from build123d import *

# Parameters (mm, degrees)
CROQUIS1_R              = 4.1
SALIENTE_EXTRUIR1_DEPTH = 0.75


with BuildPart() as part:
    # Croquis1 → Saliente-Extruir1 (new, symmetric)
    with BuildSketch(Plane(origin=(0, 0, 0), x_dir=(1, 0, 0), z_dir=(0, 1, 0))):
        with Locations(Location((0, 0, 0), (0, 0, 270))):
            Circle(CROQUIS1_R)
        with BuildLine():
            Line((1.724717498, -2.212701665), (2.778614602, -0.387298335))
            ThreePointArc((2.778614602, -0.387298335), (2.890446656, -0.263302793), (3.043155854, -0.195766112))
            ThreePointArc((3.043155854, -0.195766112), (3.2022214, 0), (3.043155854, 0.195766112))
            ThreePointArc((3.043155854, 0.195766112), (2.890446656, 0.263302793), (2.778614602, 0.387298335))
            Line((2.778614602, 0.387298335), (1.724717498, 2.212701665))
            ThreePointArc((1.724717498, 2.212701665), (1.673250235, 2.371548836), (1.691116353, 2.537567222))
            ThreePointArc((1.691116353, 2.537567222), (1.6011107, 2.773205081), (1.352039501, 2.733333333))
            ThreePointArc((1.352039501, 2.733333333), (1.217196421, 2.634851628), (1.053897104, 2.6))
            Line((1.053897104, 2.6), (-1.053897104, 2.6))
            ThreePointArc((-1.053897104, 2.6), (-1.217196421, 2.634851628), (-1.352039501, 2.733333333))
            ThreePointArc((-1.352039501, 2.733333333), (-1.6011107, 2.773205081), (-1.691116353, 2.537567222))
            ThreePointArc((-1.691116353, 2.537567222), (-1.673250235, 2.371548836), (-1.724717498, 2.212701665))
            Line((-1.724717498, 2.212701665), (-2.778614602, 0.387298335))
            ThreePointArc((-2.778614602, 0.387298335), (-2.890446656, 0.263302793), (-3.043155854, 0.195766112))
            ThreePointArc((-3.043155854, 0.195766112), (-3.2022214, 0), (-3.043155854, -0.195766112))
            ThreePointArc((-3.043155854, -0.195766112), (-2.890446656, -0.263302793), (-2.778614602, -0.387298335))
            Line((-2.778614602, -0.387298335), (-1.724717498, -2.212701665))
            ThreePointArc((-1.724717498, -2.212701665), (-1.673250235, -2.371548836), (-1.691116353, -2.537567222))
            ThreePointArc((-1.691116353, -2.537567222), (-1.6011107, -2.773205081), (-1.352039501, -2.733333333))
            ThreePointArc((-1.352039501, -2.733333333), (-1.217196421, -2.634851628), (-1.053897104, -2.6))
            Line((-1.053897104, -2.6), (1.053897104, -2.6))
            ThreePointArc((1.053897104, -2.6), (1.217196421, -2.634851628), (1.352039501, -2.733333333))
            ThreePointArc((1.352039501, -2.733333333), (1.6011107, -2.773205081), (1.691116353, -2.537567222))
            ThreePointArc((1.691116353, -2.537567222), (1.673250235, -2.371548836), (1.724717498, -2.212701665))
        make_face(mode=Mode.SUBTRACT)
    extrude(amount=SALIENTE_EXTRUIR1_DEPTH, both=True)


solid = part.part
CAD build for the part. Positions are in the model's coordinates, mm. A direction names the side the tool comes from. Give positions to 0.01 mm unless a question says otherwise; leave off trailing zeros. Write each loop counter-clockwise with the first axis right and the second up, starting at its lowest first coordinate (ties: lowest second). Pieces come first, ordered by that corner, then holes. Notation, with made-up numbers: (81, 53) - (105, 53) arc R12 cw to (105, 70) - close; hole circle Ø8 at (40.25, -10.75). An arc over 180 degrees is marked (long way). Put each result on its own line as item: value.
(1) Tool access for faces 1 (the flat face through (-2.244, 0.01, -1.313)), 2 (the flat face through (0, -0.75, 3)): list every direction of +Z, -Z, +X, -X, +Y, -Y with a clear straight run to the whole face (end or side of a thin tool).
Working result:
face 1: +Y, -Y
face 2: +Z, -Z, +X, -X, -Y
(2) Saw through at B-B (z = 0). List the corners of the cut face in (x, y).
Working result:
outline: (-4.1, -0.75) - (-3.2, -0.75) - (-3.2, 0.75) - (-4.1, 0.75) - close; (3.2, -0.75) - (4.1, -0.75) - (4.1, 0.75) - (3.2, 0.75) - close
(3) Pull direction X, two halves, no side cores. Call faces 3 (the flat face through (0, 0.75, 3)), 4 (the flat face through (2.259, 0.01, -1.287)), 5 (the cylindrical face through (4.065, 0.01, -0.534)): released by +X, released by -X, zero draft, split by the parting line, or undercut.
Working result:
face 3: zero draft
face 4: undercut
face 5: split by the parting line
(4) Saw through at C-C (y = 0.2). List the corners of the cut face in (x, z), then the cut area to 3 significant figures.
Working result:
outline: circle Ø8.2 at (0, 0); hole (-3.04, -0.2) arc R0.4 cw to (-2.78, -0.39) - (-1.72, -2.21) arc R0.4 cw to (-1.69, -2.54) arc R0.2 ccw to (-1.35, -2.73) arc R0.4 cw to (-1.05, -2.6) - (1.05, -2.6) arc R0.4 cw to (1.35, -2.73) arc R0.2 ccw to (1.69, -2.54) arc R0.4 cw to (1.72, -2.21) - (2.78, -0.39) arc R0.4 cw to (3.04, -0.2) arc R0.2 ccw to (3.04, 0.2) arc R0.4 cw to (2.78, 0.39) - (1.72, 2.21) arc R0.4 cw to (1.69, 2.54) arc R0.2 ccw to (1.35, 2.73) arc R0.4 cw to (1.05, 2.6) - (-1.05, 2.6) arc R0.4 cw to (-1.35, 2.73) arc R0.2 ccw to (-1.69, 2.54) arc R0.4 cw to (-1.72, 2.21) - (-2.78, 0.39) arc R0.4 cw to (-3.04, 0.2) arc R0.2 ccw to start
area: 28.8 mm^2
(5) Saw through at A-A (x = 0). List the corners of the cut face in (y, z).
Working result:
outline: (-0.75, -4.1) - (0.75, -4.1) - (0.75, -2.6) - (-0.75, -2.6) - close; (-0.75, 2.6) - (0.75, 2.6) - (0.75, 4.1) - (-0.75, 4.1) - close
(6) Wall check: L1, parallel to X at y = 0.05, z = 0; L2, parallel to X at y = 0.1, z = 1.25; L3, parallel to Z at x = -1.25, y = -0.2. Give the ranges that are in metal, low to high.
Working result:
L1: -4.1 to -3.2, 3.2 to 4.1
L2: -3.9 to -2.28, 2.28 to 3.9
L3: -3.9 to -2.65, 2.65 to 3.9
(7) Saw through at D-D (z = 3.5). List the corners of the cut face in (x, y).
Working result:
outline: (-2.14, -0.75) - (2.14, -0.75) - (2.14, 0.75) - (-2.14, 0.75) - close
